Could you check a few things on this model? Use its own coordinates, in mm. Coordinates: 2 decimals unless noted, no trailing zeros. Loops run counter-clockwise (first coordinate to the right, second up) from the corner with the lowest first, then second, coordinate; pieces in that order, holes last. Notation, with made-up numbers: (39, -10) -> (44, -10) arc R27 cw to (44, 13) -> close; hole circle Ø2 at (-3.75, -16). An arc over 180 degrees is marked (long way). One line per question, with ' | ' between items.
Autodesk Inventor part; units mm, degrees
ref_plane "YZ Plane" through (0, 0, 0) normal (1, 0, 0) x (0, 1, 0)
ref_plane "XZ Plane" through (0, 0, 0) normal (0, 1, 0) x (-1, 0, 0)
ref_plane "XY Plane" through (0, 0, 0) normal (0, 0, 1) x (1, 0, 0)
sketch "Sketch1" plane through (0, 0, 0) normal (0, 1, 0) x (-1, 0, 0)
  line L0 (70, 41.6667) -> (-50, 41.6667)
  line L1 (-50, 41.6667) -> (-50, -58.3333)
  line L2 (-50, -58.3333) -> (70, -58.3333)
  line L3 (70, -58.3333) -> (70, 41.6667)
  point P0 (0, 0)
  dimension "d0" = 100
  dimension "d1" = 120
  dimension "d2" = 70
  dimension "d3" = 41.6667
extrude "Extrusion1" add sketch "Sketch1" along normal blind 10
sketch "Sketch2" plane through (0, 10, 0) normal (0, 1, 0) x (1, 0, 0)
  circle A0 centre (-40, 0) radius 3.5
  circle A1 centre (-55, 0) radius 3.5
  line L0 (-70, 58.3333) -> (-70, -41.6667)
  point P0 (0, 0)
  dimension "d6" = 7
  dimension "d7" = 7
  dimension "d8" = 30
  dimension "d9" = 15
  dimension "d12" = 15
  dimension "d13" = 40
extrude "Extrusion2" cut sketch "Sketch2" against normal blind 5
thread "Thread1"
thread "Thread2"
properties part number "Load cell support" material "Stainless Steel"
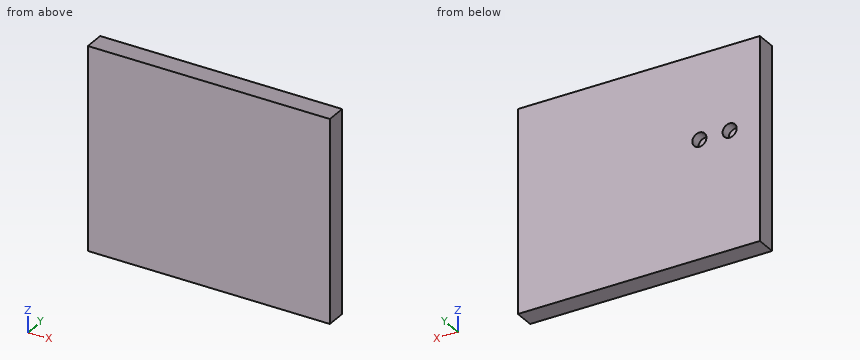
1) If we section it at B-B on x = -55: Please give me the cut outline in (y, z).
Data:
outline: (0, -58.33) -> (10, -58.33) -> (10, -3.5) -> (5, -3.5) -> (5, 3.5) -> (10, 3.5) -> (10, 41.67) -> (0, 41.67) -> close
2) I need wall thicknesses on line 1 along X through (y, z) = (6.75, 0); line 2 along Z through (x, y) = (-55, 6.4); line 3 along X through (y, z) = (7, 3). Which ranges of each line are inside material? Lowest first, please. Write a range as from..to.
Data:
line 1: -70..-58.5, -51.5..-43.5, -36.5..50 | line 2: -58.33..-3.5, 3.5..41.67 | line 3: -70..-56.8, -53.2..-41.8, -38.2..50
3) I'm going to push a flat-ended pin straight in: pin 1 Ø2 at (x, z) = (-53.5, -1.5) entering from +Y. Where does the tip first touch, or does it pass through?
Data:
pin 1: y = 5
4) If we section it at A-A on z = 0: Please give me the cut outline in (x, y), and give its area (3 significant figures).
Data:
outline: (-70, 0) -> (50, 0) -> (50, 10) -> (-36.5, 10) -> (-36.5, 5) -> (-43.5, 5) -> (-43.5, 10) -> (-51.5, 10) -> (-51.5, 5) -> (-58.5, 5) -> (-58.5, 10) -> (-70, 10) -> close | area: 1,130 mm²
